Read the model definition and answer for the solid it produces. Units are mm, in the model's axes. Face numbers are marked on the shaded views. A direction names the side the tool comes from. Give positions to 0.01 mm unless a question says otherwise; leave off trailing zeros. Write each loop counter-clockwise with the first axis right and the second up, starting at its lowest first coordinate (ties: lowest second). Pieces come first, ordered by that corner, then holes. Notation, with made-up numbers: (79.25, 60.25) - (132.25, 60.25) arc R17 cw to (132.25, 91.25) - close; hole circle Ø6 at (48.5, -32). An arc over 180 degrees is marked (long way). Answer as a JSON object with one key per item and string values. Group by question number.
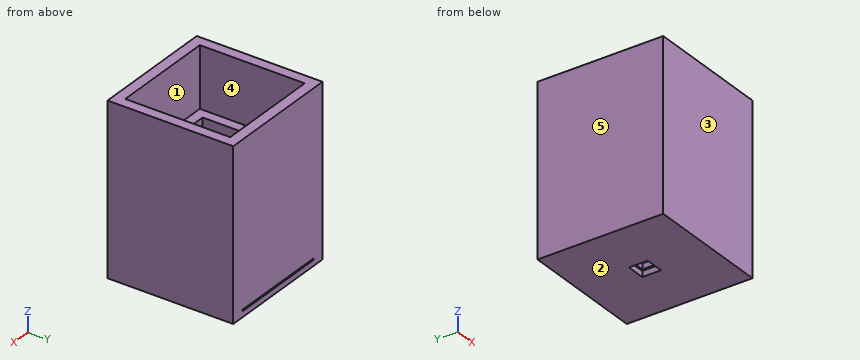
```python
from build123d import *

# Parameters (mm, degrees)
BOSS_EXTRUDE1_DEPTH      = 76.2
BOSS_EXTRUDE1_DEPTH_BACK = 6.35
SKETCH1_W                = 61.468
SKETCH1_H                = 61.468
SKETCH1_3_W              = 41.656
SKETCH1_3_H              = 41.656
CUT_EXTRUDE1_DEPTH       = 88.724554784
SKETCH2_W                = 51.308
SKETCH2_H                = 51.308
CUT_EXTRUDE2_DEPTH       = 69.511409218
SKETCH5_W                = 9.144
SKETCH5_H                = 9.144
CUT_EXTRUDE3_DEPTH       = 94.293408192
SKETCH6_W                = 48.768
SKETCH6_H                = 0.762
CUT_EXTRUDE4_DEPTH       = 55.118


with BuildPart() as part:
    # Sketch1 → Boss-Extrude1 (new, two sides: drawn at the far end of the back side and taken through both)
    with BuildSketch(Plane.XY.offset(-BOSS_EXTRUDE1_DEPTH_BACK)):
        Rectangle(SKETCH1_W, SKETCH1_H)
    extrude(amount=BOSS_EXTRUDE1_DEPTH + BOSS_EXTRUDE1_DEPTH_BACK)

    # Sketch1<3> → Cut-Extrude1 (cut, through all)
    with BuildSketch(Plane.XY):
        Rectangle(SKETCH1_3_W, SKETCH1_3_H)
    extrude(amount=CUT_EXTRUDE1_DEPTH, mode=Mode.SUBTRACT)

    # Sketch2 → Cut-Extrude2 (cut, through all)
    with BuildSketch(Plane.XY.offset(46.609)):
        Rectangle(SKETCH2_W, SKETCH2_H)
    extrude(amount=CUT_EXTRUDE2_DEPTH, mode=Mode.SUBTRACT)

    # Sketch5 → Cut-Extrude3 (cut, through all)
    with BuildSketch(Plane(origin=(0, 0, -6.35), x_dir=(-1, 0, 0), z_dir=(0, 0, -1))):
        Rectangle(SKETCH5_W, SKETCH5_H)
    extrude(amount=-CUT_EXTRUDE3_DEPTH, mode=Mode.SUBTRACT)

    # Sketch6 → Cut-Extrude4 (cut)
    with BuildSketch(Plane(origin=(0, 30.734, 0), x_dir=(1, 0, 0), z_dir=(0, 1, 0))):
        with Locations((0, 3.175)):
            Rectangle(SKETCH6_W, SKETCH6_H)
    extrude(amount=-CUT_EXTRUDE4_DEPTH, mode=Mode.SUBTRACT)


solid = part.part
```
1) Which of the six approach directions +Z, -Z, +X, -X, +Y, -Y give full straight-line access (tool end or side, diameter ignored) to the marked faces 1 and 2?
2) Find section D-D, the plane x = -18.5. Write down the section's boundary in (y, z), and give its area (3 significant figures).
3) Find the intervals of material crossed by line 1 (Z direction, x = 17.5, y = -1.5); line 2 (Y direction, x = -6, z = 20), in increasing order. Write a range as [from, to].
4) Find section C-C, the plane y = 2.5. Write down the section's boundary in (x, z), and give its area (3 significant figures).
5) Find section B-B, the plane x = 3.5. Write down the section's boundary in (y, z).
6) Flat-ended cylindrical pins translate along their axes: pin 1 Ø10 at (x, y) = (-8.5, 10) entering from +Z; pin 2 Ø8 at (x, y) = (18.5, -15) entering from +Z. Find the tip coordinate at first contact, or state that the pin passes through.
7) Find section A-A, the plane z = 10. Write down the section's boundary in (x, y), and give its area (3 significant figures).
8) For a pull along Y with two mould halves and no side action, classify the marked faces 3, 4 and 5 as released by +Y, released by -Y, zero draft, split by the parting line, or undercut.
Values follow:
{
 "1": {"face 1": "+Z", "face 2": "-Z, +X, -X, +Y, -Y"},
 "2": {"outline": "(-30.73, -6.35) - (30.73, -6.35) - (30.73, -3.56) - (-24.38, -3.56) - (-24.38, -2.79) - (30.73, -2.79) - (30.73, 76.2) - (25.65, 76.2) - (25.65, 46.61) - (20.83, 46.61) - (20.83, 0) - (-20.83, 0) - (-20.83, 46.61) - (-25.65, 46.61) - (-25.65, 76.2) - (-30.73, 76.2) - close", "area": "1,570 mm2"},
 "3": {"line 1": "z = [-6.35, -3.56], [-2.79, 0]", "line 2": "y = [-30.73, -20.83], [20.83, 30.73]"},
 "4": {"outline": "(-30.73, -6.35) - (-4.57, -6.35) - (-4.57, -3.56) - (-24.38, -3.56) - (-24.38, -2.79) - (-4.57, -2.79) - (-4.57, 0) - (-20.83, 0) - (-20.83, 46.61) - (-25.65, 46.61) - (-25.65, 76.2) - (-30.73, 76.2) - close; (4.57, -6.35) - (30.73, -6.35) - (30.73, 76.2) - (25.65, 76.2) - (25.65, 46.61) - (20.83, 46.61) - (20.83, 0) - (4.57, 0) - (4.57, -2.79) - (24.38, -2.79) - (24.38, -3.56) - (4.57, -3.56) - close", "area": "1,530 mm2"},
 "5": {"outline": "(-30.73, -6.35) - (-4.57, -6.35) - (-4.57, -3.56) - (-24.38, -3.56) - (-24.38, -2.79) - (-4.57, -2.79) - (-4.57, 0) - (-20.83, 0) - (-20.83, 46.61) - (-25.65, 46.61) - (-25.65, 76.2) - (-30.73, 76.2) - close; (4.57, -6.35) - (30.73, -6.35) - (30.73, -3.56) - (4.57, -3.56) - close; (4.57, -2.79) - (30.73, -2.79) - (30.73, 76.2) - (25.65, 76.2) - (25.65, 46.61) - (20.83, 46.61) - (20.83, 0) - (4.57, 0) - close"},
 "6": {"pin 1": "stops at z = 0", "pin 2": "stops at z = 46.61"},
 "7": {"outline": "(-30.73, -30.73) - (30.73, -30.73) - (30.73, 30.73) - (-30.73, 30.73) - close; hole (-20.83, -20.83) - (20.83, -20.83) - (20.83, 20.83) - (-20.83, 20.83) - close", "area": "2,040 mm2"},
 "8": {"face 3": "released by -Y", "face 4": "undercut", "face 5": "zero draft"}
}
